Design review of the part shown in the three views and the two pictorial views. Dimensions are in mm from the part's minimum x, y and z. A direction names the side the tool comes from. Give positions to 0.01 mm unless a question says otherwise; leave off trailing zeros. Loops run counter-clockwise (first coordinate to the right, second up) from the corner with the lowest first, then second, coordinate; pieces in that order, holes last.
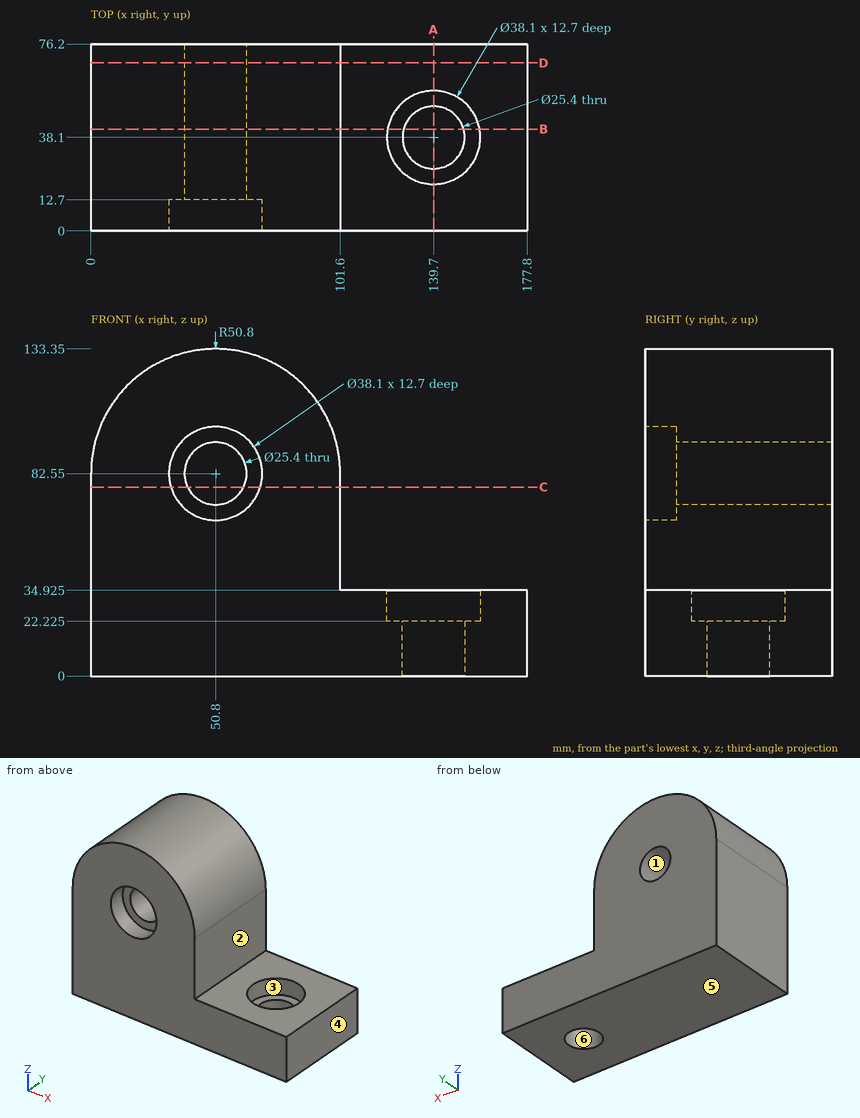
Q1. For pin 1 Ø12 at (x, y) = (129, 13) entering from +Z (3 decimals); pin 2 Ø12 at (x, y) = (26.5, 9.5) entering from +Z; pin 3 Ø11.5 at (x, y) = (132, 44) entering from +Z (3 decimals), all flat-tipped, find the tip position at first contact; note any pin that passes through.
Answers:
pin 1: stops at z = 34.925
pin 2: stops at z = 129.94
pin 3: stops at z = 22.225
Q2. Consider section D-D on y = 68.5. Give the boundary of the cut face in (x, z) (3 decimals).
Answers:
outline: (0, 0) - (177.8, 0) - (177.8, 34.925) - (101.6, 34.925) - (101.6, 82.55) arc R50.8 ccw to (0, 82.55) - close; hole circle Ø25.4 at (50.8, 82.55)
Q3. Consider section C-C on z = 77. Give the boundary of the cut face in (x, y).
Answers:
outline: (0, 0) - (32.58, 0) - (32.58, 12.7) - (39.38, 12.7) - (39.38, 76.2) - (0, 76.2) - close; (62.22, 12.7) - (69.02, 12.7) - (69.02, 0) - (101.6, 0) - (101.6, 76.2) - (62.22, 76.2) - close
Q4. Consider section B-B on y = 41.5. Give the boundary of the cut face in (x, z) (3 decimals).
Answers:
outline: (0, 0) - (127.464, 0) - (127.464, 22.225) - (120.956, 22.225) - (120.956, 34.925) - (101.6, 34.925) - (101.6, 82.55) arc R50.8 ccw to (0, 82.55) - close; (151.936, 0) - (177.8, 0) - (177.8, 34.925) - (158.444, 34.925) - (158.444, 22.225) - (151.936, 22.225) - close; hole circle Ø25.4 at (50.8, 82.55)
Q5. Machinability: for the marked faces 1, 2 and 3, which of the approach directions +Z, -Z, +X, -X, +Y, -Y give a long, thin tool a straight path to every point of the face, cutting with its end or side? Answer none if there is none.
Answers:
face 1: +Y, -Y
face 2: +Z, +X, +Y, -Y
face 3: +Z
Q6. Consider section A-A on x = 139.7. Give the boundary of the cut face in (y, z) (3 decimals).
Answers:
outline: (0, 0) - (25.4, 0) - (25.4, 22.225) - (19.05, 22.225) - (19.05, 34.925) - (0, 34.925) - close; (50.8, 0) - (76.2, 0) - (76.2, 34.925) - (57.15, 34.925) - (57.15, 22.225) - (50.8, 22.225) - close
Q7. For probe 1 along Z at (x, y) = (50.8, 6.75); probe 2 along Z at (x, y) = (50.8, 53.5); probe 3 along Y at (x, z) = (38.5, 87), list the stretches that pass through material, from the lowest coordinate up.
Answers:
probe 1: z = 0 to 63.5, 101.6 to 133.35
probe 2: z = 0 to 69.85, 95.25 to 133.35
probe 3: y = 12.7 to 76.2
Q8. Mouldability with a two-part tool opening along X and no side actions: class the marked faces 4, 5 and 6 as +X half, -X half, draft (parallel to the pull), parting line (faces both ways), or undercut.
Answers:
face 4: +X half
face 5: draft
face 6: undercut
